Read the model definition and answer for the solid it produces. Units are mm, in the model's axes. Face numbers are marked on the shaded views. Coordinates: 2 decimals unless noted, no trailing zeros. Loops run counter-clockwise (first coordinate to the right, second up) from the corner with the lowest first, then second, coordinate; pieces in that order, holes last. Notation, with made-up numbers: M -25.75,-34 L 11.25,-34 A28 ccw 11.25,-3 Z; hole C -2,82.5 d9. An arc over 180 degrees is marked long. Use one line per item in the form item = value. Start each with the question number.
1. The part is cut by section C-C (y = 38.5). Give the vertices of the cut face in (x, z), plus the area to 3 significant figures.
2. For a pull along X with two mould halves and no side action, classify the marked faces 1, 2 and 3 as released by +X, released by -X, zero draft, split by the parting line, or undercut.
3. The part is cut by section D-D (z = 60.5). Give the vertices of the cut face in (x, y), plus the area to 3 significant figures.
4. Flat-ended cylindrical pins translate along their axes: pin 1 (1 mm diameter, centred on y = 5, z = 17.5, fed in from +X); pin 2 (1 mm diameter, centred on x = 24.5, y = -15.5, fed in from -Z); pin 3 (12 mm diameter, centred on x = -6, y = -22.5, fed in from -Z). Find the tip coordinate at first contact, or state that the pin passes through.
5. Find the intervals of material crossed by probe 1 along Y at (x, z) = (-15, 17); probe 2 along Z at (x, y) = (14, -18); probe 3 along Y at (x, z) = (16, 12), in increasing order. Write a range as [from, to].
6. The part is cut by section A-A (z = 8). Give the vertices of the cut face in (x, y), plus the area to 3 significant figures.
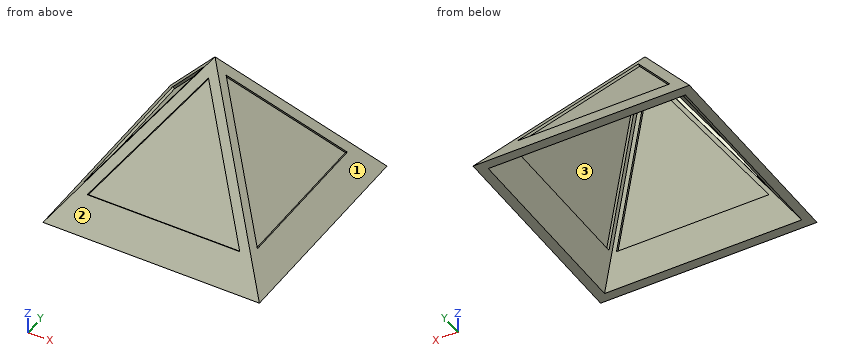
from build123d import *

# Parameters (mm, degrees)
F3_W      = 90
F3_H      = 90
F8_W      = 82
F8_H      = 82
F14_DEPTH = 1
F15_START = -2
F15_DEPTH = 3
F17_DEPTH = 1
F18_START = -2
F18_DEPTH = 3
F20_DEPTH = 1
F21_START = -2
F21_DEPTH = 3
F23_DEPTH = 1
F24_START = -2
F24_DEPTH = 3


with BuildPart() as f6:
    # F3 (on Top) → F6 section 0
    with BuildSketch(Plane.XY, mode=Mode.PRIVATE) as f6_s0:
        Rectangle(F3_W, F3_H)
    loft([f6_s0.sketch, Vertex(0, 0, 63.6396103068)])

    # F8 (on Top) → F10 section 0
    with BuildSketch(Plane.XY, mode=Mode.PRIVATE) as f10_s0:
        Rectangle(F8_W, F8_H)
    loft([f10_s0.sketch, Vertex(0, 0, 57.9827560573)], mode=Mode.SUBTRACT)

    # F13 (on offset) → F14 (cut)
    with BuildSketch(Plane(origin=(0, -30, 21.2132034356), x_dir=(1, 0, 0), z_dir=(0, -0.8164965809, 0.5773502692))):
        Polygon((31.7209438086, -10.9807621135), (0, 43.9615242271), (-31.7209438086, -10.9807621135), align=None)
    extrude(amount=-F14_DEPTH, mode=Mode.SUBTRACT)

    # F13 (on offset) → F15 (cut)
    with BuildSketch(Plane(origin=(0, -30, 21.2132034356), x_dir=(1, 0, 0), z_dir=(0, -0.8164965809, 0.5773502692)).offset(F15_START)):
        Polygon((31.7209438086, -10.9807621135), (0, 43.9615242271), (-31.7209438086, -10.9807621135), align=None)
    extrude(amount=-F15_DEPTH, mode=Mode.SUBTRACT)

    # F16 (on offset) → F17 (cut)
    with BuildSketch(Plane(origin=(-30, 0, 21.2132034356), x_dir=(0, -1, 0), z_dir=(-0.8164965809, 0, 0.5773502692))):
        Polygon((31.7209438086, -10.9807621135), (0, 43.9615242271), (-31.7209438086, -10.9807621135), align=None)
    extrude(amount=-F17_DEPTH, mode=Mode.SUBTRACT)

    # F16 (on offset) → F18 (cut)
    with BuildSketch(Plane(origin=(-30, 0, 21.2132034356), x_dir=(0, -1, 0), z_dir=(-0.8164965809, 0, 0.5773502692)).offset(F18_START)):
        Polygon((31.7209438086, -10.9807621135), (0, 43.9615242271), (-31.7209438086, -10.9807621135), align=None)
    extrude(amount=-F18_DEPTH, mode=Mode.SUBTRACT)

    # F19 (on face) → F20 (cut)
    with BuildSketch(Plane(origin=(0, 30, 21.2132034356), x_dir=(-1, 0, 0), z_dir=(0, 0.8164965809, 0.5773502692))):
        Polygon((31.7209438086, -10.9807621135), (0, 43.9615242271), (-31.7209438086, -10.9807621135), align=None)
    extrude(amount=-F20_DEPTH, mode=Mode.SUBTRACT)

    # F19 (on face) → F21 (cut)
    with BuildSketch(Plane(origin=(0, 30, 21.2132034356), x_dir=(-1, 0, 0), z_dir=(0, 0.8164965809, 0.5773502692)).offset(F21_START)):
        Polygon((31.7209438086, -10.9807621135), (0, 43.9615242271), (-31.7209438086, -10.9807621135), align=None)
    extrude(amount=-F21_DEPTH, mode=Mode.SUBTRACT)

    # F22 (on face) → F23 (cut)
    with BuildSketch(Plane(origin=(30, 0, 21.2132034356), x_dir=(0, 1, 0), z_dir=(0.8164965809, 0, 0.5773502692))):
        Polygon((31.7209438086, -10.9807621135), (0, 43.9615242271), (-31.7209438086, -10.9807621135), align=None)
    extrude(amount=-F23_DEPTH, mode=Mode.SUBTRACT)

    # F22 (on face) → F24 (cut)
    with BuildSketch(Plane(origin=(30, 0, 21.2132034356), x_dir=(0, 1, 0), z_dir=(0.8164965809, 0, 0.5773502692)).offset(F24_START)):
        Polygon((31.7209438086, -10.9807621135), (0, 43.9615242271), (-31.7209438086, -10.9807621135), align=None)
    extrude(amount=-F24_DEPTH, mode=Mode.SUBTRACT)


solid = f6.part
Computed values:
q1.outline = M -45,0 L -41,0 L -38.5,3.54 L 38.5,3.54 L 41,0 L 45,0 L 38.5,9.19 L -38.5,9.19 Z
q1.area = 486 mm²
q2.face_1 = released by +X
q2.face_2 = zero draft
q2.face_3 = undercut
q3.outline = M -2.22,-2.22 L 2.22,-2.22 L 2.22,2.22 L -2.22,2.22 Z
q3.area = 19.7 mm²
q4.pin_1 = 31.75
q4.pin_2 = 24.82
q4.pin_3 = 19.87
q5.probe_1 = [-31.75, -30.53], [30.53, 31.75]
q5.probe_2 = [34.72, 36.45], [36.87, 38.18]
q5.probe_3 = [-36.51, -35.99], [-35.29, -34.07], [34.07, 35.29], [35.99, 36.51]
q6.outline = M -39.34,-39.34 L 39.34,-39.34 L 39.34,39.34 L -39.34,39.34 Z; hole M -35.34,-35.34 L 35.34,-35.34 L 35.34,35.34 L -35.34,35.34 Z
q6.area = 1,190 mm²
